For this review, take the finished solid that the model builds, in its own axes (mm). Coordinates: 2 decimals unless noted, no trailing zeros. Order: outer loops, then holes, each group sorted by start corner. A loop starts at its lowest first (then second) coordinate and runs counter-clockwise, first axis right, second up. Notation, with made-up numbers: (50, -9.75) -> (55, -9.75) arc R13 ccw to (55, -2.75) -> close; hole circle Ø1 at (-9.75, 18.5). An arc over 180 degrees is marked (long way). Answer as a JSON object with one key per item and string values. Group by question number.
1) Draft analysis for pull direction Z (two halves, no side actions). For faces 1 (the cylindrical face through (-21.18, 2.817, 23.865)), 2 (the flat face through (17, 3, -50.927)), 3 (the cylindrical face through (17.17, 2.82, 26.18)), 4 (the flat face through (17, 3, 34.925)), state which applies: +Z half, -Z half, draft (parallel to the pull), parting line (faces both ways), or undercut.
2) Add section D-D, the plane x = 0. Write out the cut boundary in (y, z) (3 decimals), then the cut area to 4 significant figures.
3) Wall thickness on L1, parallel to Z at x = 41.91, y = 3.9 (3 decimals); L2, parallel to X at y = 5.3, z = -42; L3, parallel to X at y = 3.15, z = -15.5: over which ranges is each line inside the solid? List them lowest first.
4) For pin 1 (2 mm diameter, centred on x = 41.91, z = 24.765, fed in from +Y), flat-tipped, find the tip position at first contact; note if it passes through.
5) Add section B-B, the plane x = -13.97. Write out the cut boundary in (y, z) (3 decimals), then the cut area to 3 significant figures.
6) Add section C-C, the plane z = 13. Write out the cut boundary in (x, y) (3 decimals).
7) Add section A-A, the plane z = 0. Write out the cut boundary in (x, y) (3 decimals).
from build123d import *

# Parameters (mm, degrees)
SKETCH1_W                = 94.488
SKETCH1_H                = 85.852
SKETCH1_R                = 9.779
SKETCH1_R_2              = 10.668
BOSS_EXTRUDE1_DEPTH      = 5.715
M3_CLEARANCE_HOLE1_D     = 3.7
M3_CLEARANCE_HOLE1_DEPTH = 25.4
M3_CLEARANCE_HOLE1_TIP   = 1.111592145


with BuildPart() as part:
    # Sketch1 → Boss-Extrude1 (new body)
    with BuildSketch(Plane(origin=(0, 0, 0), x_dir=(1, 0, 0), z_dir=(0, 1, 0))):
        with Locations((18.034, 8.001)):
            Rectangle(SKETCH1_W, SKETCH1_H)
        with Locations(Location((-13.97, 16.002, 0), (0, 0, 270))):
            Circle(SKETCH1_R, mode=Mode.SUBTRACT)
        with Locations(Location((13.97, 16.002, 0), (0, 0, 90))):
            Circle(SKETCH1_R_2, mode=Mode.SUBTRACT)
        with Locations(Location((13.97, -16.002, 0), (0, 0, 270))):
            Circle(SKETCH1_R_2, mode=Mode.SUBTRACT)
        with Locations(Location((-13.97, -16.002, 0), (0, 0, 90))):
            Circle(SKETCH1_R_2, mode=Mode.SUBTRACT)
    extrude(amount=BOSS_EXTRUDE1_DEPTH)

    # M3 Clearance Hole1
    with Locations(Plane(origin=(0, 5.715, 0), x_dir=(1, 0, 0), z_dir=(0, 1, 0))):
        with Locations((41.656, 42.037), (41.91, -24.765), (-17.78, 33.147), (41.656, 5.207), (41.656, 28.067), (0, 0)):
            Hole(M3_CLEARANCE_HOLE1_D / 2, depth=M3_CLEARANCE_HOLE1_DEPTH)
            with Locations((0, 0, -(M3_CLEARANCE_HOLE1_DEPTH + M3_CLEARANCE_HOLE1_TIP / 2))):  # 118° drill point
                Cone(0, M3_CLEARANCE_HOLE1_D / 2, M3_CLEARANCE_HOLE1_TIP, mode=Mode.SUBTRACT)


solid = part.part
Output values:
{
 "1": {"face 1": "undercut", "face 2": "-Z half", "face 3": "undercut", "face 4": "+Z half"},
 "2": {"outline": "(0, -50.927) -> (5.715, -50.927) -> (5.715, -1.85) -> (0, -1.85) -> close; (0, 1.85) -> (5.715, 1.85) -> (5.715, 34.925) -> (0, 34.925) -> close", "area": "469.5 mm²"},
 "3": {"L1": "z = -50.927 to -43.869, -40.205 to -29.899, -26.235 to -7.039, -3.375 to 22.915, 26.615 to 34.925", "L2": "x = -29.21 to 39.81, 43.51 to 65.28", "L3": "x = -29.21 to -23.74, -4.2 to 3.31, 24.63 to 65.28"},
 "4": {"pin 1": "passes through"},
 "5": {"outline": "(0, -50.927) -> (5.715, -50.927) -> (5.715, -25.781) -> (0, -25.781) -> close; (0, -6.223) -> (5.715, -6.223) -> (5.715, 5.334) -> (0, 5.334) -> close; (0, 26.67) -> (5.715, 26.67) -> (5.715, 34.925) -> (0, 34.925) -> close", "area": "257 mm²"},
 "6": {"outline": "(-29.21, 0) -> (-24.207, 0) -> (-24.207, 5.715) -> (-29.21, 5.715) -> close; (-3.733, 0) -> (3.733, 0) -> (3.733, 5.715) -> (-3.733, 5.715) -> close; (24.207, 0) -> (65.278, 0) -> (65.278, 5.715) -> (24.207, 5.715) -> close"},
 "7": {"outline": "(-29.21, 0) -> (-1.85, 0) -> (-1.85, 5.715) -> (-29.21, 5.715) -> close; (1.85, 0) -> (65.278, 0) -> (65.278, 5.715) -> (1.85, 5.715) -> close"}
}
